```python
from build123d import *

# Parameters (mm, degrees)
SKETCH1_R                 = 78.359
SKETCH1_R_2               = 76.2
BOSS_EXTRUDE1_DEPTH       = 914.4
SKETCH2_W                 = 3.175
SKETCH2_H                 = 194.31
FIN_SLOTS_DEPTH           = 922.090454712
CIRPATTERN1_COUNT         = 4
SKETCH3_R                 = 3.175
RAIL_BUTTONS_DEPTH        = 922.090454712
SKETCH2_4_R               = 1.0922
SHEAR_SCREW_HOLES_DEPTH   = 922.090454829
SHEAR_SCREW_PATTERN_COUNT = 4


with BuildPart() as part:
    # Sketch1 → Boss-Extrude1 (new body)
    with BuildSketch(Plane(origin=(0, 0, 0), x_dir=(1, 0, 0), z_dir=(0, 1, 0))):
        with Locations(Location((0, 0, 0), (0, 0, 270))):
            Circle(SKETCH1_R)
        with Locations(Location((0, 0, 0), (0, 0, 270))):
            Circle(SKETCH1_R_2, mode=Mode.SUBTRACT)
    extrude(amount=BOSS_EXTRUDE1_DEPTH)

    # Sketch2 → Fin Slots (cut, through all)
    with BuildSketch(Plane(origin=(0, 0, 0), x_dir=(0, 0, -1), z_dir=(1, 0, 0))):
        with Locations((0, 106.045)):
            Rectangle(SKETCH2_W, SKETCH2_H)
    fin_slots = extrude(amount=-FIN_SLOTS_DEPTH, mode=Mode.SUBTRACT)

    # CirPattern1: Fin Slots ×4 about axis
    cirpattern1_axis = Axis((0, 0, 0), (0, 1, 0))
    for i in range(1, CIRPATTERN1_COUNT):
        add(fin_slots.rotate(cirpattern1_axis, i * 360 / CIRPATTERN1_COUNT), mode=Mode.SUBTRACT)

    # Sketch3 → Rail Buttons (cut, through all)
    with BuildSketch(Plane(origin=(0, 0, 0), x_dir=(0.7071067811865477, 0, -0.7071067811865475), z_dir=(0.7071067811865475, 0, 0.7071067811865477))):
        with Locations((0, 127)):
            Circle(SKETCH3_R)
        with Locations((0, 742.95)):
            Circle(SKETCH3_R)
    extrude(amount=-RAIL_BUTTONS_DEPTH, mode=Mode.SUBTRACT)

    # Sketch2_4 → Shear Screw Holes (cut, through all)
    with BuildSketch(Plane(origin=(0, 0, 0), x_dir=(0, 0, -1), z_dir=(1, 0, 0))):
        with Locations((0, 800.1)):
            Circle(SKETCH2_4_R)
    shear_screw_holes = extrude(amount=-SHEAR_SCREW_HOLES_DEPTH, mode=Mode.SUBTRACT)

    # Shear Screw Pattern: Shear Screw Holes ×4 about axis
    shear_screw_pattern_axis = Axis((0, 914.4, 0), (0, -1, 0))
    for i in range(1, SHEAR_SCREW_PATTERN_COUNT):
        add(shear_screw_holes.rotate(shear_screw_pattern_axis, i * 360 / SHEAR_SCREW_PATTERN_COUNT), mode=Mode.SUBTRACT)


solid = part.part
```
Input: part model. Units: mm. Frame: model coordinates. Give positions to 0.01 mm unless a question says otherwise; leave off trailing zeros. Write each loop counter-clockwise with the first axis right and the second up, starting at its lowest first coordinate (ties: lowest second). Pieces come first, ordered by that corner, then holes. Notation, with made-up numbers: (57, 10) - (106, 10) arc R35 cw to (106, 47) - close; hole circle Ø3 at (79, 24). An arc over 180 degrees is marked (long way). Write item = value, one per line. Start each with the question number.
1. Section query C-C, the plane y = 657.5. Output: boundary loops of the cut face in (x, z), then the cut area to 3 significant figures.
2. Section query B-B, the plane z = 22. Output: boundary loops of the cut face in (x, y).
3. Mould query, pull axis X, two halves, no side actions, for faces 1 (the cylindrical face through (-46.367, 450.799, -60.47)), 2 (the flat face through (-75, 0, 17)), 3 (the cylindrical face through (23.54, 450.8, 74.74)). Classes: released by +X, released by -X, zero draft, split by the parting line, or undercut.
4. Ray query, L1, parallel to Y at x = 0, z = 77; L2, parallel to X at y = 450, z = 0; L3, parallel to X at y = 861.5, z = -4.5. Return the intervals inside material, ascending.
5. First-contact query: pin 1 Ø1.5 at (x, y) = (-41, 712) entering from +Z; pin 2 Ø1 at (y, z) = (119, -48) entering from +X; pin 3 Ø3 at (x, y) = (-12, 817) entering from +Z. Flat tips, straight axial feed; report the tip coordinate or a pass-through.
6. Section query A-A, the plane x = -66.5. Output: boundary loops of the cut face in (y, z), then the cut area to 3 significant figures.
Check sheet entries:
q1.outline = circle Ø156.72 at (0, 0); hole circle Ø152.4 at (0, 0)
q1.area = 1,050 mm2
q2.outline = (-75.21, 0) - (-72.96, 0) - (-72.96, 914.4) - (-75.21, 914.4) - close; (72.96, 0) - (75.21, 0) - (75.21, 914.4) - (72.96, 914.4) - close
q3.face_1 = undercut
q3.face_2 = zero draft
q3.face_3 = split by the parting line
q4.L1 = 0 to 8.89, 203.2 to 799.01, 801.19 to 914.4
q4.L2 = -78.36 to -76.2, 76.2 to 78.36
q4.L3 = -78.23 to -76.07, 76.07 to 78.23
q5.pin_1 = 67.23
q5.pin_2 = 62.32
q5.pin_3 = 77.65
q6.outline = (0, -41.45) - (914.4, -41.45) - (914.4, -37.2) - (0, -37.2) - close; (0, 37.2) - (914.4, 37.2) - (914.4, 41.45) - (0, 41.45) - close
q6.area = 7,760 mm2
